Geometry: see drawing. Coordinates: mm, zero at the bounding-box minimum. A direction names the side the tool comes from. Give positions to 0.01 mm unless a question says otherwise; leave off trailing zeros. Write each loop counter-clockwise with the first axis right and the second up, starting at its lowest first coordinate (ties: lowest second). Pieces come first, ordered by that corner, then holes. Notation, with made-up numbers: (-37, 55.5) -> (4, 55.5) arc R28 cw to (4, 76.5) -> close; hole circle Ø10 at (65, 51.25). An arc over 180 degrees is marked (long way). Write item = value, one per line.
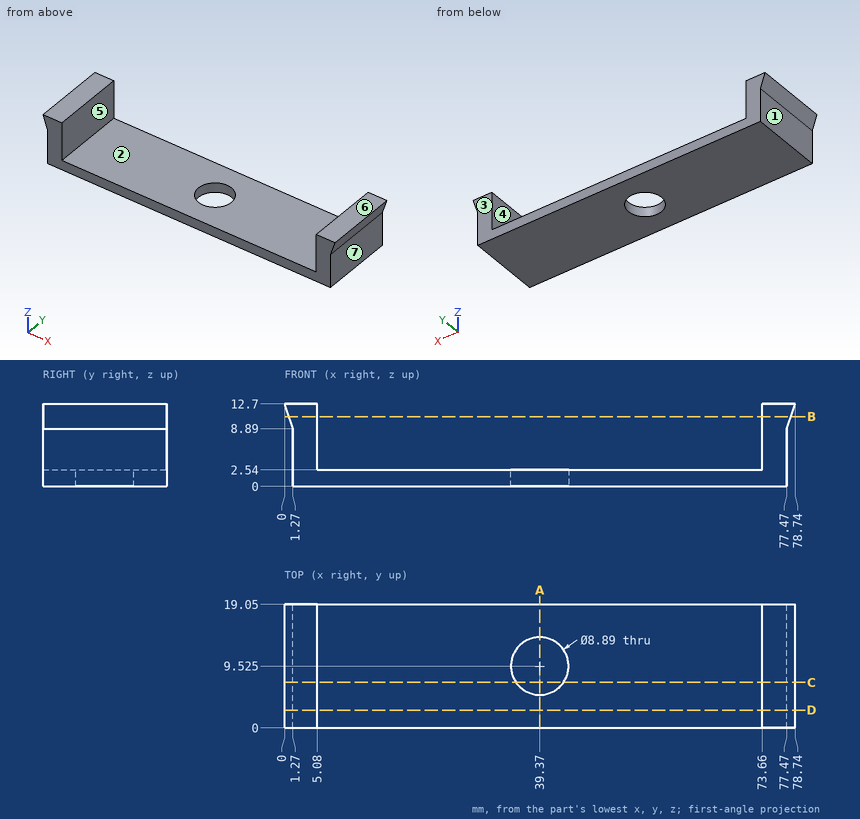
(1) Section query C-C (y = 7). Return loops of the section in (x, z), plus the area to 3 significant figures.
Values follow:
outline = (0, 12.7) -> (1.27, 8.89) -> (1.27, 0) -> (35.71, 0) -> (35.71, 2.54) -> (5.08, 2.54) -> (5.08, 12.7) -> close; (43.03, 0) -> (77.47, 0) -> (77.47, 8.89) -> (78.74, 12.7) -> (73.66, 12.7) -> (73.66, 2.54) -> (43.03, 2.54) -> close
area = 257 mm2
(2) Material intervals for line 1 (X direction, y = 5.5, z = 3.5); line 2 (Z direction, x = 27, y = 15); line 3 (Y direction, x = 39.37, z = 0.95), sorted ascending.
Values follow:
line_1 = 1.27 to 5.08, 73.66 to 77.47
line_2 = 0 to 2.54
line_3 = 0 to 5.08, 13.97 to 19.05
(3) Section query B-B (z = 10.75). Return loops of the section in (x, y), plus the area to 3 significant figures.
Values follow:
outline = (0.65, 0) -> (5.08, 0) -> (5.08, 19.05) -> (0.65, 19.05) -> close; (73.66, 0) -> (78.09, 0) -> (78.09, 19.05) -> (73.66, 19.05) -> close
area = 169 mm2
(4) Access query for the marked faces 5, 6 and 7. Directions: +Z, -Z, +X, -X, +Y, -Y. A direction counts if a zero-diameter tool reaches every point of the face in a straight line with its end or side. Return the directions, or none.
Values follow:
face_5 = +Z, +Y, -Y
face_6 = +Z, +X, -X, +Y, -Y
face_7 = -Z, +X, +Y, -Y
(5) Pull-direction query (X, two-part tool) for the marked faces 1, 2, 3 and 4; classes: pulls with the +X half, pulls with the -X half, needs draft (parallel to the pull), parting line crosses it, or undercut.
Values follow:
face_1 = pulls with the -X half
face_2 = undercut
face_3 = needs draft
face_4 = undercut
(6) Section query A-A (x = 39.37). Return loops of the section in (y, z), plus the area to 3 significant figures.
Values follow:
outline = (0, 0) -> (5.08, 0) -> (5.08, 2.54) -> (0, 2.54) -> close; (13.97, 0) -> (19.05, 0) -> (19.05, 2.54) -> (13.97, 2.54) -> close
area = 25.8 mm2
(7) First-contact query: pin 1 (2.5 mm diameter, centred on y = 7.5, z = 6.5, fed in from +X); pin 2 (10 mm diameter, centred on x = 29, y = 16, fed in from +Z); pin 3 (2 mm diameter, centred on y = 13, z = 9.5, fed in from +X); pin 4 (7 mm diameter, centred on x = 39.37, y = 9.525, fed in from -Z). Flat tips, straight axial feed; report the tip coordinate or a pass-through.
Values follow:
pin_1 = 77.47
pin_2 = 2.54
pin_3 = 78.01
pin_4 = through
(8) Section query D-D (y = 2.75). Return loops of the section in (x, z).
Values follow:
outline = (0, 12.7) -> (1.27, 8.89) -> (1.27, 0) -> (77.47, 0) -> (77.47, 8.89) -> (78.74, 12.7) -> (73.66, 12.7) -> (73.66, 2.54) -> (5.08, 2.54) -> (5.08, 12.7) -> close
